Here's how the part is built. I have some questions about the finished solid (model axes, mm). Face numbers are marked on the shaded views. A direction names the side the tool comes from. Round coordinates to 2 decimals unless told otherwise and drop trailing zeros. Write each loop counter-clockwise with the first axis right and the second up, starting at its lowest first coordinate (ties: lowest second). Pieces come first, ordered by that corner, then holes. Notation, with made-up numbers: (73, 30.25) -> (82, 30.25) arc R31 ccw to (82, 59.25) -> close; hole circle Ø10 at (-21.5, 21). An arc over 180 degrees is marked (long way). Answer as CSV lines item,"result".
```python
from build123d import *

# Parameters (mm, degrees)
BOSS_EXTRUDE1_DEPTH            = 114.3
CUT_EXTRUDE2_DEPTH             = 161.602521773
CUT_EXTRUDE1_DEPTH             = 158.090324336
FILLET1_R                      = 45.72
SHELL1_T                       = -3.175
SKETCH6_W                      = 6.35
SKETCH6_H                      = 26.924
CUT_EXTRUDE3_REACH             = 145.438
F_1_16_0_457_DOWEL_HOLE1_D     = 11.6078
F_1_16_0_457_DOWEL_HOLE1_DEPTH = 6.35
FILLET2_R                      = 6.35


with BuildPart() as part:
    # Sketch1 → Boss-Extrude1 (new body)
    with BuildSketch(Plane(origin=(0, 0, 0), x_dir=(1, 0, 0), z_dir=(0, 1, 0))):
        Polygon((0, 0), (27.1, 83.2), (49.1, 83.2), (76.2, 0), align=None)
    extrude(amount=BOSS_EXTRUDE1_DEPTH)

    # Sketch5 → Cut-Extrude2 (cut, through all)
    with BuildSketch(Plane.XZ):
        Polygon((49.1, -83.2), (51.380048077, -76.2), (24.819951923, -76.2), (27.1, -83.2), align=None)
    extrude(amount=-CUT_EXTRUDE2_DEPTH, mode=Mode.SUBTRACT)

    # Sketch2 → Cut-Extrude1 (cut, through all)
    with BuildSketch(Plane(origin=(0, 0, 0), x_dir=(0, 0, -1), z_dir=(1, 0, 0))):
        Polygon((0, 114.3), (76.2, 38.1), (76.2, 114.3), align=None)
        Polygon((0, 88.9), (76.2, 12.7), (76.2, 0), (0, 0), align=None)
    extrude(amount=CUT_EXTRUDE1_DEPTH, mode=Mode.SUBTRACT)

    # Fillet1
    fillet1_edges = [part.edges().sort_by_distance(p)[0] for p in [
        (38.1, 38.1, -76.2),
    ]]
    fillet(fillet1_edges, radius=FILLET1_R)

    # Shell1
    shell1_openings = [part.faces().sort_by_distance(p)[0] for p in [
        (38.1, 56.934937611, -31.965062389),
    ]]
    offset(amount=SHELL1_T, openings=shell1_openings, kind=Kind.INTERSECTION)

    # Sweep1: sweep along a path in Sketch7
    with BuildLine(Plane.ZY.offset(-38.1)) as sweep1_path:
        Line((-35.849182435, 73.960689504), (-35.849182435, 23.160689504))
    # Sketch6 → Sweep1 (sweep)
    with BuildSketch(Plane(origin=(0, 54.90493597, -54.90493597), x_dir=(1, 0, 0), z_dir=(0, -0.7071067811865517, 0.7071067811865434))):
        with Locations((38.1, 26.94890509)):
            Rectangle(SKETCH6_W, SKETCH6_H)
    sweep(path=sweep1_path.line)

    # Sketch11 → Cut-Extrude3 (cut, up to next)
    with BuildSketch(Plane.ZY.offset(-34.925), mode=Mode.PRIVATE) as cut_extrude3_sk1:
        Polygon((-26.330110947, 42.210689504), (-45.368253924, 42.210689504), (-45.368253924, 13.641618016), (-26.330110947, 32.679760992), align=None)
    cut_extrude3_tool1 = extrude(cut_extrude3_sk1.sketch, amount=-CUT_EXTRUDE3_REACH, mode=Mode.PRIVATE) & part.part
    add(cut_extrude3_tool1.solids().sort_by_distance((34.925, 31.892927, -37.434707))[0], mode=Mode.SUBTRACT)

    # 1/16 (0.457) Dowel Hole1
    with Locations(Plane.ZY.offset(-34.925)):
        with Locations((-35.849182435, 51.729760992)):
            Hole(F_1_16_0_457_DOWEL_HOLE1_D / 2, depth=F_1_16_0_457_DOWEL_HOLE1_DEPTH)

    # Fillet2
    fillet2_edges = [part.edges().sort_by_distance(p)[0] for p in [
        (38.1, 42.210689504, -26.330110947),
        (38.1, 42.210689504, -45.368253924),
    ]]
    fillet(fillet2_edges, radius=FILLET2_R)


solid = part.part
```
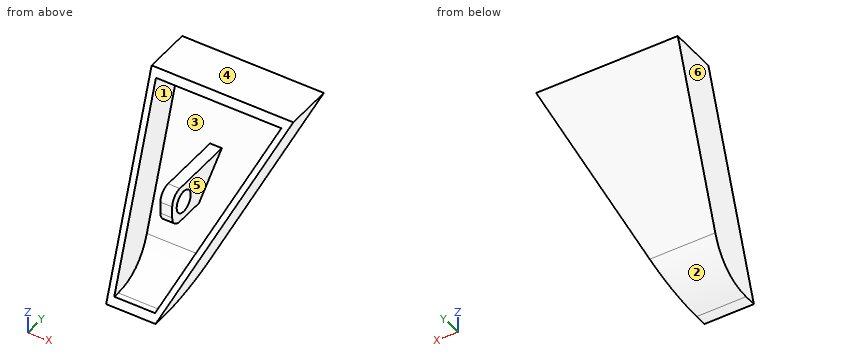
1. Suppose I cut it at C-C on x = 39. Please give me the cut outline in (y, z) (3 decimals).
Numbers:
outline,"(12.7, -76.2) -> (19.162, -76.2) arc R45.72 ccw to (51.491, -62.809) -> (114.3, 0) -> (88.9, 0) -> (85.725, -3.175) -> (106.635, -3.175) -> (83.48, -26.33) -> (48.561, -26.33) arc R6.35 ccw to (42.211, -32.68) -> (42.211, -39.018) arc R6.35 ccw to (48.561, -45.368) -> (64.442, -45.368) -> (49.246, -60.564) arc R42.545 cw to (19.162, -73.025) -> (15.875, -73.025) -> close; hole circle Ø11.608 at (51.73, -35.849)"
2. If we mould it in two halves opening along Z, with no side actions, what happens to the marked faces 3, 4, 5 and 6? For each: released by +Z, released by -Z, zero draft, split by the parting line, or undercut.
Numbers:
face 3,"undercut"
face 4,"released by +Z"
face 5,"zero draft"
face 6,"released by -Z"
3. On a 3-axis mill with a long thin cutter (end or side, diameter ignored), from which of +Z, -Z, +X, -X, +Y, -Y can I reach the whole of each face in a straight line? I mean the marked faces 1 and 2. Say none if no direction works.
Numbers:
face 1,"-Y"
face 2,"-Z, +X, -X, +Y"
4. For pin 1 Ø7 at (x, z) = (37.5, -36.5) entering from -Y; pin 2 Ø21 at (y, z) = (63, -32) entering from +X; pin 3 Ø4 at (x, z) = (28.5, -52) entering from +Y; pin 4 Ø2 at (x, y) = (41.5, 91) entering from +Z, each with a flat end and sliding along its axis, tell me the tip position at first contact or that it passes through.
Numbers:
pin 1,"stops at y = 42.21"
pin 2,"stops at x = 68.98"
pin 3,"stops at y = 64.3"
pin 4,"stops at z = 0"
5. If I drill on line 1 (X direction, y = 56.5, z = -42) (3 decimals); line 2 (X direction, y = 84, z = -17); line 3 (X direction, y = 84, z = -23.5), over which ranges is the centre line in solid material (lowest first)?
Numbers:
line 1,"x = 13.68 to 17.019, 34.925 to 41.275, 59.181 to 62.52"
line 2,"x = 5.54 to 8.88, 67.32 to 70.66"
line 3,"x = 7.65 to 10.99, 65.21 to 68.55"
6. Suppose I cut it at A-A on y = 54. Please give me the cut outline in (x, z) (3 decimals).
Numbers:
outline,"(11.368, -34.9) -> (19.641, -60.3) -> (56.559, -60.3) -> (64.832, -34.9) -> (61.493, -34.9) -> (54.682, -55.81) -> (21.518, -55.81) -> (14.707, -34.9) -> close; (34.925, -45.368) -> (41.275, -45.368) -> (41.275, -41.191) -> (34.925, -41.191) -> close; (34.925, -30.508) -> (41.275, -30.508) -> (41.275, -26.33) -> (34.925, -26.33) -> close"
7. Suppose I cut it at D-D on z = -20. Please give me the cut outline in (x, y), and give its area (3 significant figures).
Numbers:
outline,"(6.51, 68.9) -> (9.85, 68.9) -> (9.85, 89.81) -> (66.35, 89.81) -> (66.35, 68.9) -> (69.69, 68.9) -> (69.69, 94.3) -> (6.51, 94.3) -> close"
area,"423 mm^2"
8. Suppose I cut it at B-B on x = 7.5. Please give me the cut outline in (y, z) (3 decimals), and give its area (3 significant figures).
Numbers:
outline,"(65.874, -23.026) -> (91.274, -23.026) -> (114.3, 0) -> (88.9, 0) -> (85.725, -3.175) -> (106.635, -3.175) -> (97.036, -12.774) -> (76.126, -12.774) -> close"
area,"384 mm^2"
